from build123d import *

# Parameters (mm, degrees)
BOSS_EXTRUDE1_START   = 600
SKETCH1_R             = 57.281017464
SKETCH1_R_2           = 38.771715285
BOSS_EXTRUDE1_DEPTH   = 293
SKETCH1_R_3           = 35.256926628
SKETCH1_R_4           = 25.147423748
BOSS_EXTRUDE1_2_DEPTH = 293
SKETCH1_R_5           = 31.428515318
SKETCH1_R_6           = 24.521075722
BOSS_EXTRUDE1_3_DEPTH = 293
SKETCH1_R_7           = 43.796557911
SKETCH1_R_8           = 32.254492843
BOSS_EXTRUDE1_4_DEPTH = 293
SKETCH2_W             = 616.707969139
SKETCH2_H             = 76.195303947
SKETCH2_H_2           = 103.48726304
BOSS_EXTRUDE2_DEPTH   = 34
SKETCH6_R             = 9.313662058
CUT_EXTRUDE3_DEPTH    = 126


with BuildPart() as part:
    # Sketch1 → Boss-Extrude1 (new body)
    with BuildSketch(Plane.XY.offset(427.014108562).offset(BOSS_EXTRUDE1_START)):
        with Locations((1173.639225527, -317.201613393)):
            Circle(SKETCH1_R)
        with Locations((1173.639225527, -317.201613393)):
            Circle(SKETCH1_R_2, mode=Mode.SUBTRACT)
    extrude(amount=BOSS_EXTRUDE1_DEPTH)



with BuildPart() as body_2:
    # Sketch1 → Boss-Extrude1 2 (new body)
    with BuildSketch(Plane.XY.offset(427.014108562).offset(BOSS_EXTRUDE1_START)):
        with Locations((491.765116758, -317.201613393)):
            Circle(SKETCH1_R_3)
        with Locations((491.765116758, -317.201613393)):
            Circle(SKETCH1_R_4, mode=Mode.SUBTRACT)
    extrude(amount=BOSS_EXTRUDE1_2_DEPTH)


with BuildPart() as body_3:
    # Sketch1 → Boss-Extrude1 3 (new body)
    with BuildSketch(Plane.XY.offset(427.014108562).offset(BOSS_EXTRUDE1_START)):
        with Locations((491.765116758, -2112.860849235)):
            Circle(SKETCH1_R_5)
        with Locations((491.765116758, -2112.860849235)):
            Circle(SKETCH1_R_6, mode=Mode.SUBTRACT)
    extrude(amount=BOSS_EXTRUDE1_3_DEPTH)


with BuildPart() as body_4:
    # Sketch1 → Boss-Extrude1 4 (new body)
    with BuildSketch(Plane.XY.offset(427.014108562).offset(BOSS_EXTRUDE1_START)):
        with Locations((1173.639225527, -2112.860849235)):
            Circle(SKETCH1_R_7)
        with Locations((1173.639225527, -2112.860849235)):
            Circle(SKETCH1_R_8, mode=Mode.SUBTRACT)
    extrude(amount=BOSS_EXTRUDE1_4_DEPTH)


with BuildPart() as part_1:
    add(part.part)

    add(body_2.part)  # Boss-Extrude2 merges body 2

    add(body_3.part)  # Boss-Extrude2 merges body 3

    add(body_4.part)  # Boss-Extrude2 merges body 4
    # Sketch2 → Boss-Extrude2 (add)
    with BuildSketch(Plane(origin=(0, 0, 1027.014108562), x_dir=(-1, 0, 0), z_dir=(0, 0, -1))):
        Polygon((-1134.867510242, 91.617150216), (-1134.867510242, 172.765208514), (-1033.166693927, 91.617150216), (-1033.166693927, -2363.997444221), (-1134.867510242, -2363.997444221), align=None)
        Polygon((-518.159541103, -2363.997444221), (-617.883714932, -2363.997444221), (-617.883714932, 88.905828795), (-518.159541103, 172.765208514), (-518.159541103, 88.905828795), align=None)
        with Locations((-826.513525673, -2116.408610896)):
            Rectangle(SKETCH2_W, SKETCH2_H)
        with Locations((-826.513525673, -335.838828239)):
            Rectangle(SKETCH2_W, SKETCH2_H_2)
    extrude(amount=-BOSS_EXTRUDE2_DEPTH)

    # Sketch6 → Cut-Extrude3 (cut)
    with BuildSketch(Plane(origin=(0, -284.095196719, 0), x_dir=(1, 0, 0), z_dir=(0, 1, 0))):
        with Locations(Location((838.898443774, -1047.155157013, 0), (0, 0, 270))):
            Circle(SKETCH6_R)
    extrude(amount=-CUT_EXTRUDE3_DEPTH, mode=Mode.SUBTRACT)


solid = part_1.part
Read the model definition and answer for the solid it produces. Units are mm, in the model's axes. A direction names the side the tool comes from. Round coordinates to 2 decimals unless told otherwise and drop trailing zeros. Write each loop counter-clockwise with the first axis right and the second up, starting at its lowest first coordinate (ties: lowest second). Pieces come first, ordered by that corner, then holes.
Q1. Find section A-A on z = 1214.5. Determine the outline of the cut face in (x, y).
Values:
outline: circle Ø70.51 at (491.77, -317.2); circle Ø62.86 at (491.77, -2112.86); circle Ø114.56 at (1173.64, -317.2); circle Ø87.59 at (1173.64, -2112.86); hole circle Ø50.29 at (491.77, -317.2); hole circle Ø49.04 at (491.77, -2112.86); hole circle Ø77.54 at (1173.64, -317.2); hole circle Ø64.51 at (1173.64, -2112.86)
Q2. A tool of negligible diameter and unlimited length cuts with its end or side. For faces 3 (the face through (568.72, 130.25, 1043.78)), 4 (the face through (1170.2, -2145.1, 1320.014)), from which of +Z, -Z, +X, -X, +Y, -Y can it reach the whole face along a straight path? Write none if from no direction.
Values:
face 3: +Z, -Z, +Y
face 4: +Z, +X, -X, +Y, -Y
Q3. Find section B-B on x = 764. Determine the outline of the cut face in (y, z).
Values:
outline: (-2154.51, 1027.01) - (-2078.31, 1027.01) - (-2078.31, 1061.01) - (-2154.51, 1061.01) - close; (-387.58, 1027.01) - (-284.1, 1027.01) - (-284.1, 1061.01) - (-387.58, 1061.01) - close
Q4. The mould has two halves that part along X. Classify faces 1 (the face through (475, -2131, 1320.014)), 2 (the face through (460.367, -2111.479, 1171.463)): released by +X, released by -X, zero draft, split by the parting line, or undercut.
Values:
face 1: zero draft
face 2: undercut
Q5. Find section C-C on y = -1508.5. Determine the outline of the cut face in (x, z), and give its area (3 significant figures).
Values:
outline: (518.16, 1027.01) - (617.88, 1027.01) - (617.88, 1061.01) - (518.16, 1061.01) - close; (1033.17, 1027.01) - (1134.87, 1027.01) - (1134.87, 1061.01) - (1033.17, 1061.01) - close
area: 6,850 mm2
Q6. Flat-ended cylindrical pins translate along their axes: P1, Ø17, axis at y = -49, z = 1037.5, coming from the -X side; P2, Ø17, axis at y = -2270.5, z = 1047.5, coming from the +X side. Find the tip coordinate at first contact, or state that the pin passes through.
Values:
P1: stops at x = 518.16
P2: stops at x = 1134.87
Q7. Straight lines are drawn through the part: line 1 (Y direction, x = 493, z = 1261.5); line 2 (Y direction, x = 495.5, z = 1106); line 3 (X direction, y = -312.5, z = 1120). For each, find the intervals that lie inside material, in ascending order.
Values:
line 1: y = -2144.27 to -2137.35, -2088.37 to -2081.46, -352.44 to -342.32, -292.08 to -281.97
line 2: y = -2144.07 to -2137.1, -2088.63 to -2081.66, -352.26 to -342.07, -292.33 to -282.14
line 3: x = 456.82 to 467.06, 516.47 to 526.71, 1116.55 to 1135.15, 1212.12 to 1230.73
